Build history of the part. All positions in model axes, mm. Face numbers are marked on the shaded views. A direction names the side the tool comes from. Round coordinates to 2 decimals unless told otherwise and drop trailing zeros. Loops run counter-clockwise (first coordinate to the right, second up) from the corner with the lowest first, then second, coordinate; pieces in that order, holes last. Notation, with made-up numbers: (-32.75, 25.25) - (21.25, 25.25) arc R19 cw to (21.25, 50.25) - close; hole circle Ø11 at (75, 73.5). An arc over 180 degrees is marked (long way). Use a Markdown table: item, result.
from build123d import *

# Parameters (mm, degrees)
SKETCH1_W           = 42
SKETCH1_H           = 42
SKETCH1_R           = 1.5
SKETCH1_R_2         = 11
BOSS_EXTRUDE1_DEPTH = 40.3
SKETCH1_3_R         = 1.5
CUT_EXTRUDE1_DEPTH  = 5
SKETCH1_4_R         = 11
BOSS_EXTRUDE2_DEPTH = 1.8
CHAMFER1_SIZE       = 4.5
SKETCH2_R           = 2.5
BOSS_EXTRUDE3_DEPTH = 20.75


with BuildPart() as part:
    # Sketch1 → Boss-Extrude1 (new body)
    # profile 1 of 6: a face of its own
    with BuildSketch(Plane.XY):
        Rectangle(SKETCH1_W, SKETCH1_H)
        with Locations((-15.5, 15.5)):
            Circle(SKETCH1_R, mode=Mode.SUBTRACT)
        with Locations((-15.5, -15.5)):
            Circle(SKETCH1_R, mode=Mode.SUBTRACT)
        with Locations((15.5, -15.5)):
            Circle(SKETCH1_R, mode=Mode.SUBTRACT)
        with Locations((15.5, 15.5)):
            Circle(SKETCH1_R, mode=Mode.SUBTRACT)
        Circle(SKETCH1_R_2, mode=Mode.SUBTRACT)
    # profile 2 of 6: a face of its own
    with BuildSketch(Plane.XY):
        with Locations((-15.5, -15.5)):
            Circle(SKETCH1_R)
    # profile 3 of 6: a face of its own
    with BuildSketch(Plane.XY):
        with Locations((15.5, -15.5)):
            Circle(SKETCH1_R)
    # profile 4 of 6: a face of its own
    with BuildSketch(Plane.XY):
        Circle(SKETCH1_R_2)
    # profile 5 of 6: a face of its own
    with BuildSketch(Plane.XY):
        with Locations((-15.5, 15.5)):
            Circle(SKETCH1_R)
    # profile 6 of 6: a face of its own
    with BuildSketch(Plane.XY):
        with Locations((15.5, 15.5)):
            Circle(SKETCH1_R)
    extrude(amount=BOSS_EXTRUDE1_DEPTH)

    # Sketch1_3 → Cut-Extrude1 (cut)
    with BuildSketch(Plane.XY):
        with Locations((15.5, 15.5)):
            Circle(SKETCH1_3_R)
        with Locations((-15.5, 15.5)):
            Circle(SKETCH1_3_R)
        with Locations((15.5, -15.5)):
            Circle(SKETCH1_3_R)
        with Locations((-15.5, -15.5)):
            Circle(SKETCH1_3_R)
    extrude(amount=CUT_EXTRUDE1_DEPTH, mode=Mode.SUBTRACT)

    # Sketch1_4 → Boss-Extrude2 (add)
    with BuildSketch(Plane.XY):
        Circle(SKETCH1_4_R)
    extrude(amount=-BOSS_EXTRUDE2_DEPTH)

    # Chamfer1
    chamfer1_edges = [part.edges().sort_by_distance(p)[0] for p in [
        (-21, -21, 20.15),
        (-21, 21, 20.15),
        (21, 21, 20.15),
        (21, -21, 20.15),
    ]]
    chamfer(chamfer1_edges, length=CHAMFER1_SIZE)

    # Sketch2 → Boss-Extrude3 (add)
    with BuildSketch(Plane(origin=(0, 0, -1.8), x_dir=(-1, 0, 0), z_dir=(0, 0, -1))):
        with Locations(Location((0, 0, 0), (0, 0, 180))):
            Circle(SKETCH2_R)
    extrude(amount=BOSS_EXTRUDE3_DEPTH)


solid = part.part
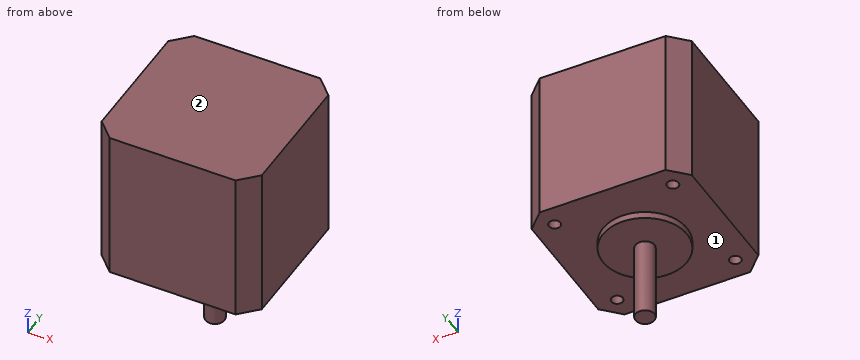
Q1. Cut at A-A, the plane x = 15.5. List the corners of the cut face in (y, z).
Results found:
| item | result |
|---|---|
| outline | (-21, 0) - (-17, 0) - (-17, 5) - (-14, 5) - (-14, 0) - (14, 0) - (14, 5) - (17, 5) - (17, 0) - (21, 0) - (21, 40.3) - (-21, 40.3) - close |
Q2. Cut at D-D, the plane y = -4.5. List the corners of the cut face in (x, z), plus the area to 3 significant figures.
Results found:
| item | result |
|---|---|
| outline | (-21, 0) - (-10.04, 0) - (-10.04, -1.8) - (10.04, -1.8) - (10.04, 0) - (21, 0) - (21, 40.3) - (-21, 40.3) - close |
| area | 1,730 mm2 |
Q3. Cut at C-C, the plane y = 0. List the corners of the cut face in (x, z).
Results found:
| item | result |
|---|---|
| outline | (-21, 0) - (-11, 0) - (-11, -1.8) - (-2.5, -1.8) - (-2.5, -22.55) - (2.5, -22.55) - (2.5, -1.8) - (11, -1.8) - (11, 0) - (21, 0) - (21, 40.3) - (-21, 40.3) - close |
Q4. Probe line 1 (Y direction, x = -15.5, z = 3.85); line 2 (Z direction, x = 7, y = 10); line 3 (Z direction, x = -2, y = 7). List the from-to ranges inside material, lowest first.
Results found:
| item | result |
|---|---|
| line 1 | y = -21 to -17, -14 to 14, 17 to 21 |
| line 2 | z = 0 to 40.3 |
| line 3 | z = -1.8 to 40.3 |
Q5. Drop flat-ended pins along their axis: pin 1 (0.9 mm diameter, centred on x = -15, y = -15, fed in from -Z); pin 2 (3.5 mm diameter, centred on x = -15.5, y = 15.5, fed in from -Z); pin 3 (1 mm diameter, centred on x = -8.5, z = -3, fed in from +Y); pin 4 (1.5 mm diameter, centred on x = 9.5, z = -2, fed in from -Y). Give the stop position or say it passes through.
Results found:
| item | result |
|---|---|
| pin 1 | stops at z = 5 |
| pin 2 | stops at z = 0 |
| pin 3 | passes through |
| pin 4 | stops at y = -6.63 |
Q6. Cut at B-B, the plane z = 7.5. List the corners of the cut face in (x, y).
Results found:
| item | result |
|---|---|
| outline | (-21, -16.5) - (-16.5, -21) - (16.5, -21) - (21, -16.5) - (21, 16.5) - (16.5, 21) - (-16.5, 21) - (-21, 16.5) - close |
Q7. Which spindle directions (+Z, -Z, +X, -X, +Y, -Y) get a long thin tool onto all of the face, cutting with end or side? Do the marked faces 1 and 2. Say none if no direction does.
Results found:
| item | result |
|---|---|
| face 1 | -Z |
| face 2 | +Z, +X, -X, +Y, -Y |
